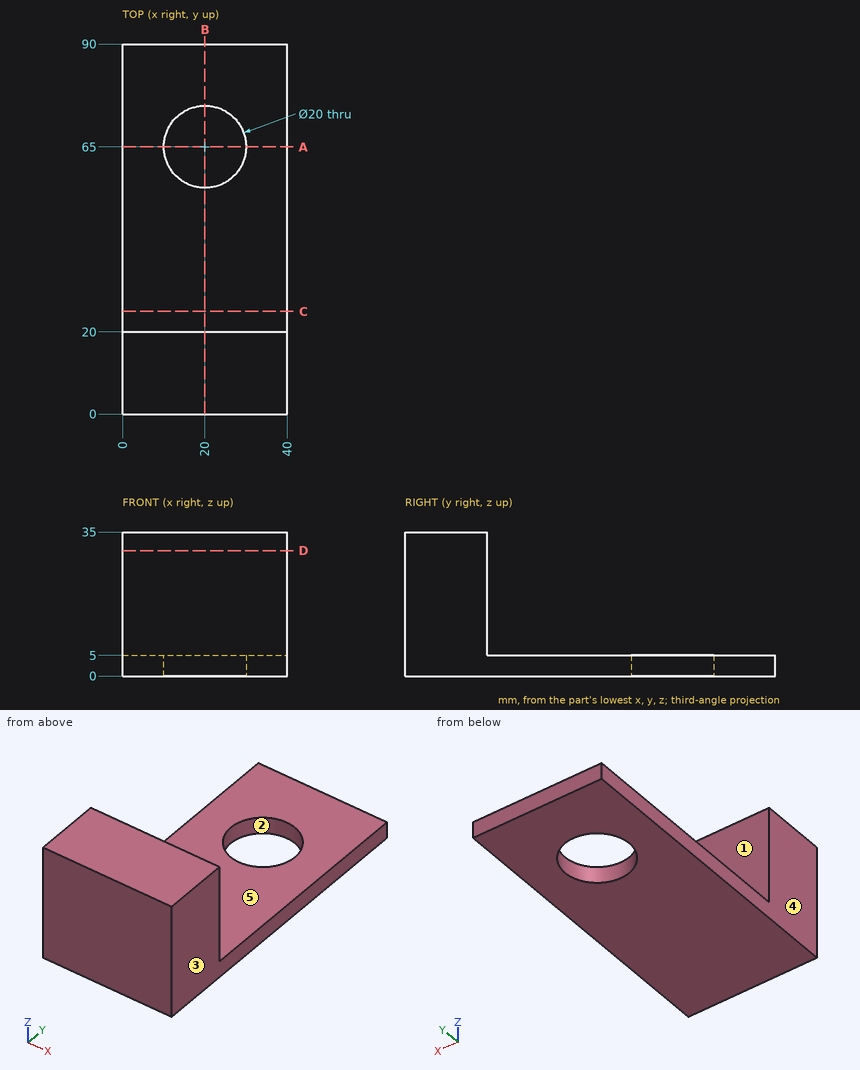
Design review of the part shown in the three views and the two pictorial views. Dimensions are in mm from the part's minimum x, y and z. A direction names the side the tool comes from. Round coordinates to 2 decimals unless told otherwise and drop trailing zeros. Write each loop counter-clockwise with the first axis right and the second up, starting at its lowest first coordinate (ties: lowest second). Pieces come first, ordered by that corner, then holes. Notation, with made-up numbers: (10, -1.5) -> (52, -1.5) arc R22 cw to (52, 36.5) -> close; hole circle Ø9 at (88, -26.5). An arc over 180 degrees is marked (long way). Use one line per item in the form item = value.
1) Take a section at D-D, the plane z = 30.5. Write out the cut boundary in (x, y), and give its area (3 significant figures).
Found:
outline = (0, 0) -> (40, 0) -> (40, 20) -> (0, 20) -> close
area = 800 mm2
2) To check wall thickness, follow L1, parallel to Y at x = 20, z = 1.85; L2, parallel to Y at x = 10, z = 26; L3, parallel to Z at x = 30, y = 31.5. State the ranges of each line that lie inside material, in increasing order. Write a range as from..to.
Found:
L1 = 0..55, 75..90
L2 = 0..20
L3 = 0..5
3) Take a section at A-A, the plane y = 65. Write out the cut boundary in (x, z), and give its area (3 significant figures).
Found:
outline = (0, 0) -> (10, 0) -> (10, 5) -> (0, 5) -> close; (30, 0) -> (40, 0) -> (40, 5) -> (30, 5) -> close
area = 100 mm2
4) Take a section at C-C, the plane y = 25. Write out the cut boundary in (x, z).
Found:
outline = (0, 0) -> (40, 0) -> (40, 5) -> (0, 5) -> close
5) Take a section at B-B, the plane x = 20. Write out the cut boundary in (y, z).
Found:
outline = (0, 0) -> (55, 0) -> (55, 5) -> (20, 5) -> (20, 35) -> (0, 35) -> close; (75, 0) -> (90, 0) -> (90, 5) -> (75, 5) -> close
6) Clearance check with flat-ended pins moving along their axes: pin 1 (6 mm diameter, centred on x = 5, y = 25.5, fed in from +Z); pin 2 (15 mm diameter, centred on x = 19.5, z = 21.5, fed in from +Y). State where each tip first meets the part, or that it passes through.
Found:
pin_1 = 5
pin_2 = 20
7) Tool access review of the marked faces 4 and 5: name each direction out of +Z, -Z, +X, -X, +Y, -Y from which nothing blocks a thin tool from reaching the whole face with its end or side.
Found:
face_4 = +Z, -Z, -X, +Y, -Y
face_5 = +Z, +X, -X, +Y
8) Mouldability with a two-part tool opening along X and no side actions: class the marked faces 1, 2 and 3 as +X half, -X half, draft (parallel to the pull), parting line (faces both ways), or undercut.
Found:
face_1 = draft
face_2 = undercut
face_3 = +X half
